from build123d import *

# Parameters (mm, degrees)
F0_W          = 215.10625
F0_H          = 55.5625
F0_R          = 3.96875
F0_R_2        = 3.571875
F0_R_3        = 11.90625
F1_DEPTH      = 6.35
F2_W          = 4.7625
F2_H          = 25.4
F3_DEPTH      = 332
F3_DEPTH_BACK = 6.351
F5_DEPTH      = 3.175
F7_DEPTH      = 4.7625
F7_DEPTH_BACK = 3.175


# Not quite as in the source:
# - an extrude ends at something that could not be found from the text; its depth is read off the source's solid


with BuildPart() as f1:
    # F0 (on Front) → F1 (new body)
    with BuildSketch(Plane.XZ):
        with Locations((107.553125, 27.78125)):
            Rectangle(F0_W, F0_H)
        with Locations((72.23125, 27.7749)):
            Circle(F0_R, mode=Mode.SUBTRACT)
        with Locations((117.475, 27.78125)):
            Circle(F0_R_2, mode=Mode.SUBTRACT)
        with Locations((161.13125, 27.78125)):
            Circle(F0_R_3, mode=Mode.SUBTRACT)
    extrude(amount=F1_DEPTH)

    # F2 (on face) → F3 (cut, two sides)
    with BuildSketch(Plane.XZ.offset(6.35)) as f3_sk:
        with Locations((28.575, 27.78125)):
            Rectangle(F2_W, F2_H)
    extrude(amount=F3_DEPTH, mode=Mode.SUBTRACT)
    extrude(f3_sk.sketch, amount=-F3_DEPTH_BACK, mode=Mode.SUBTRACT)

    # F4 (on face) → F5 (cut)
    with BuildSketch(Plane.XZ):
        with BuildLine():
            Line((57.15, 10.3124), (130.175, 10.3124))
            ThreePointArc((130.175, 10.3124), (136.9101920908, 13.1022079092), (139.7, 19.8374))
            Line((139.7, 19.8374), (139.7, 35.7124))
            ThreePointArc((139.7, 35.7124), (136.9101920908, 42.4475920908), (130.175, 45.2374))
            Line((130.175, 45.2374), (57.15, 45.2374))
            ThreePointArc((57.15, 45.2374), (50.4148079092, 42.4475920908), (47.625, 35.7124))
            Line((47.625, 35.7124), (47.625, 19.8374))
            ThreePointArc((47.625, 19.8374), (50.4148079092, 13.1022079092), (57.15, 10.3124))
        make_face()
    extrude(amount=F5_DEPTH, mode=Mode.SUBTRACT)

    # F6 (on face) → F7 (cut, two sides)
    with BuildSketch(Plane.XZ) as f7_sk:
        with BuildLine():
            Line((69.05625, 15.0749), (75.40625, 15.0749))
            ThreePointArc((75.40625, 15.0749), (76.99375, 16.6624), (75.40625, 18.2499))
            Line((75.40625, 18.2499), (69.05625, 18.2499))
            ThreePointArc((69.05625, 18.2499), (67.46875, 16.6624), (69.05625, 15.0749))
        make_face()
    extrude(amount=F7_DEPTH, mode=Mode.SUBTRACT)
    extrude(f7_sk.sketch, amount=-F7_DEPTH_BACK, mode=Mode.SUBTRACT)


solid = f1.part
Can you work these out from the model? Positions are in its coordinate system, mm. A direction names the side the tool comes from. Give positions to 0.01 mm unless a question says otherwise; leave off trailing zeros. Order: outer loops, then holes, each group sorted by start corner. A loop starts at its lowest first (then second) coordinate and runs counter-clockwise, first axis right, second up. Notation, with made-up numbers: M 59.5,78.5 L 100.5,78.5 A17 cw 100.5,96.5 Z; hole C 71.5,46.25 d8. An arc over 180 degrees is marked long. Use a Markdown table: item, result. Add a question column.
Item 1: Suppose I cut it at C-C (z = 22). List the corners of the cut face in (x, y) for me (3 decimals), then the cut area to 3 significant figures.
Item 2: Suppose I cut it at D-D (y = -1.25). Count the separate pieces of the cut face and the enclosed holes in it, then the cut area to 3 significant figures.
Item 3: Will these pins go through, and if not, where does the flat tip stop? pin 1 (1 mm diameter, centred on y = -5, z = 46.5, fed in from -X); pin 2 (1 mm diameter, centred on x = 71, z = 17, fed in from +Y); pin 3 (1 mm diameter, centred on x = 171.5, z = 27.5, fed in from +Y).
Item 4: For faces 1 (the flat face through (29, -3, 40.481)), 2 (the cylindrical face through (136.84, -1.57, 13.03)), 3 (the flat face through (0, -3, 27)), which set-ups out of +Z, -Z, +X, -X, +Y, -Y let a thin tool reach every point of the face, with its end or its side?
Item 5: We'd pull the mould along Z, two halves only. Please class faces 4 (the cylindrical face through (136.984, -1.565, 42.373)), 5 (the flat face through (106, -3, 0)), 6 (the flat face through (106, -6.35, 28)), 7 (the flat face through (106, -3, 55.562)): +Z half, -Z half, draft (parallel to the pull), parting line (faces both ways), or undercut.
Item 6: Suppose I cut it at B-B (x = 153). List the corners of the cut face in (y, z) for me, then the cut area to 3 significant figures.
Item 7: If I drill on L1, parallel to X at y = -4, z = 21; L2, parallel to X at y = -5.25, z = 18; L3, parallel to Z at x = 122, y = -0.5, over which ranges is the centre line in solid material (lowest first)? Write a range as [from, to].
Answer sheet:
| question | item | result |
|---|---|---|
| 1 | outline | M 0,-6.35 L 26.194,-6.35 L 26.194,0 L 0,0 Z; M 30.956,-6.35 L 150.723,-6.35 L 150.723,0 L 139.7,0 L 139.7,-3.175 L 47.625,-3.175 L 47.625,0 L 30.956,0 Z; M 171.54,-6.35 L 215.106,-6.35 L 215.106,0 L 171.54,0 Z |
| 1 | area | 911 mm² |
| 2 | separate pieces | 1 |
| 2 | enclosed holes | 3 |
| 2 | area | 8,250 mm² |
| 3 | pin 1 | stops at x = 0 |
| 3 | pin 2 | stops at y = -4.76 |
| 3 | pin 3 | passes through |
| 4 | face 1 | +Y, -Y |
| 4 | face 2 | +Y |
| 4 | face 3 | +Z, -Z, -X, +Y, -Y |
| 5 | face 4 | undercut |
| 5 | face 5 | -Z half |
| 5 | face 6 | draft |
| 5 | face 7 | +Z half |
| 6 | outline | M -6.35,0 L 0,0 L 0,19.08 L -6.35,19.08 Z; M -6.35,36.48 L 0,36.48 L 0,55.56 L -6.35,55.56 Z |
| 6 | area | 242 mm² |
| 7 | L1 | x = [0, 26.19], [30.96, 151.34], [170.92, 215.11] |
| 7 | L2 | x = [0, 26.19], [30.96, 154.34], [167.92, 215.11] |
| 7 | L3 | z = [0, 10.31], [45.24, 55.56] |
